Input: part model. Units: mm. Frame: model coordinates. A direction names the side the tool comes from. Round coordinates to 2 decimals unless told otherwise and drop trailing zeros. Loops run counter-clockwise (first coordinate to the right, second up) from the corner with the lowest first, then second, coordinate; pieces in that order, holes last. Notation, with made-up numbers: (-14, 9) - (12, 9) arc R12 ccw to (12, 30) - close; hole circle Ø1 at (15.25, 85). An arc over 180 degrees is marked (long way). Write each question's results on one line, items separated by ' | '.
from build123d import *

# Parameters (mm, degrees)
SKETCH1_R                = 2.25
CORNER_DEPTH             = 19
NUT_START                = -6
NUT_DEPTH                = 1.75
CHAMFER1_SIZE            = 0.5
CUT_EXTRUDE1_START       = -6
CUT_EXTRUDE1_DEPTH       = 2.5
CHAMFER1_OF_MIRROR1_SIZE = 0.5


with BuildPart() as part:
    # Sketch1 → corner (new, symmetric)
    with BuildSketch(Plane.XY):
        with BuildLine():
            Line((17.5, 2.5), (14.235015678, 5.764984322))
            ThreePointArc((14.235015678, 5.764984322), (13.988392374, 13.988392374), (5.764984322, 14.235015678))
            Line((5.764984322, 14.235015678), (2.5, 17.5))
            Line((2.5, 17.5), (0, 17.5))
            Line((0, 17.5), (0, 10))
            ThreePointArc((0, 10), (2.928932188, 2.928932188), (10, 0))
            Line((10, 0), (17.5, 0))
            Line((17.5, 0), (17.5, 2.5))
        make_face()
        with Locations((10.1, 10.1)):
            Circle(SKETCH1_R, mode=Mode.SUBTRACT)
    extrude(amount=CORNER_DEPTH, both=True)

    # Sketch4 → nut (cut, symmetric)
    with BuildSketch(Plane.XY.offset(19).offset(NUT_START)):
        Polygon((8.964337735, 14.338349272), (12.289329799, 18.716832073), (18.544552679, 12.601797863), (14.338349272, 8.964337735), (11.235662265, 5.861650728), (6.997312992, 6.997312992), (5.861650728, 11.235662265), align=None)
    nut = extrude(amount=NUT_DEPTH, both=True, mode=Mode.SUBTRACT)

    # Chamfer1
    chamfer1_edges = [part.edges().sort_by_distance(p)[0] for p in [
        (13.938348825, 14.037852483, 14.75),
        (13.938348825, 14.037852483, 11.25),
    ]]
    chamfer(chamfer1_edges, length=CHAMFER1_SIZE)

    # Sketch6 → Cut-Extrude1 (cut, symmetric)
    with BuildSketch(Plane.XY.offset(19).offset(CUT_EXTRUDE1_START)):
        Polygon((2.5, 17.5), (2.5, 14.235015678), (5.764984322, 14.235015678), align=None)
        Polygon((14.235015678, 5.764984322), (14.235015678, 2.5), (17.5, 2.5), align=None)
    cut_extrude1 = extrude(amount=CUT_EXTRUDE1_DEPTH, both=True, mode=Mode.SUBTRACT)

    # Mirror1: nut, Cut-Extrude1 across plane
    add(nut.mirror(Plane.XY), mode=Mode.SUBTRACT)
    add(cut_extrude1.mirror(Plane.XY), mode=Mode.SUBTRACT)

    # Chamfer1 of Mirror1
    chamfer1_of_mirror1_edges = [part.edges().sort_by_distance(p)[0] for p in [
        (13.938348825, 14.037852483, -14.75),
        (13.938348825, 14.037852483, -11.25),
    ]]
    chamfer(chamfer1_of_mirror1_edges, length=CHAMFER1_OF_MIRROR1_SIZE)


solid = part.part
1. Contact query for flat-ended pins moving along their axis: pin 1 (1 mm diameter, centred on x = 16, z = 12, fed in from +Y); pin 2 (2 mm diameter, centred on x = 6.5, z = 5.5, fed in from +Y); pin 3 (1 mm diameter, centred on x = 16.5, z = -13.5, fed in from +Y); pin 4 (4 mm diameter, centred on x = 10.1, y = 10.1, fed in from +Z). Output: stop coordinate, or through.
Answer:
pin 1: y = 10.17 | pin 2: y = 15.31 | pin 3: y = 2.5 | pin 4: through
2. Mould query, pull axis Z, two halves, no side actions, for faces 6 (the cylindrical face through (2.85, 3.01, 0.27)), 7 (the flat face through (9.49, 15.03, 13.03)). Classes: pulls with the +Z half, pulls with the -Z half, needs draft (parallel to the pull), parting line crosses it, or undercut.
Answer:
face 6: needs draft | face 7: undercut
3. Set-up query: faces 1 (the flat face through (17.5, 1, 0)), 2 (the flat face through (4, 14.235, -13)), 3 (the cylindrical face through (9.612, 7.904, -16.905)), 4 (the flat face through (13, 11, -14.75)), 5 (the flat face through (7.391, 12.765, 13.024)). Return all of +Z, -Z, +X, -X, +Y, -Y with unobstructed straight access to the full face (end or side cutting, diameter ignored); none if empty.
Answer:
face 1: +Z, -Z, +X, +Y, -Y | face 2: +Y | face 3: +Z, -Z | face 4: none | face 5: +X
4. Section query D-D, the plane x = 1.5. Output: boundary loops of the cut face in (y, z), plus the area to 3 significant figures.
Answer:
outline: (4.73, -19) - (17.5, -19) - (17.5, 19) - (4.73, 19) - close | area: 485 mm^2
5. Section query C-C, the plane x = 10.5. Count the separate pieces of the cut face and the enclosed holes in it, plus the area to 3 significant figures.
Answer:
separate pieces: 4 | enclosed holes: 0 | area: 391 mm^2
6. Line query: line 1 (X direction, y = 10.1, z = -3.75); line 2 (Z direction, x = 14.5, y = 13); line 3 (Z direction, x = 12.5, y = 13.75). Output: solid intervals per line, ascending. Write a range as [from, to].
Answer:
line 1: [0, 7.85], [12.35, 15.74] | line 2: [-19, -15.01], [-10.99, 10.99], [15.01, 19] | line 3: [-19, -14.75], [-11.25, 11.25], [14.75, 19]
7. Section query B-B, the plane y = 3.5. Output: boundary loops of the cut face in (x, z).
Answer:
outline: (2.4, -19) - (16.5, -19) - (16.5, -15.5) - (14.24, -15.5) - (14.24, -10.5) - (16.5, -10.5) - (16.5, 10.5) - (14.24, 10.5) - (14.24, 15.5) - (16.5, 15.5) - (16.5, 19) - (2.4, 19) - close
